Check sheet for the modelled part. Datum: model origin and axes. Units: mm. A direction names the side the tool comes from. Coordinates: 2 decimals unless noted, no trailing zeros. Loops run counter-clockwise (first coordinate to the right, second up) from the corner with the lowest first, then second, coordinate; pieces in that order, holes last. Notation, with made-up numbers: M 43.25,47.5 L 52.25,47.5 A11 ccw 52.25,59.5 Z; hole C 54,37.25 d7. An arc over 180 degrees is marked long. Return JSON: item names as keys, results as strings.
from build123d import *

# Parameters (mm, degrees)
SKETCH_R      = 2.5
PAD_DEPTH     = 65
SKETCH001_W   = 8
SKETCH001_H   = 6
SKETCH001_W_2 = 7
POCKET_DEPTH  = 1.5
CHAMFER_SIZE  = 0.3


with BuildPart() as part:
    # Sketch → Pad (new body)
    with BuildSketch(Plane.YZ):
        Circle(SKETCH_R)
    extrude(amount=PAD_DEPTH)

    # Sketch001 → Pocket (cut)
    with BuildSketch(Plane.XY.offset(3)):
        with Locations((20.5, 0)):
            Rectangle(SKETCH001_W, SKETCH001_H)
        with Locations((45.5, 0)):
            Rectangle(SKETCH001_W_2, SKETCH001_H)
    extrude(amount=-POCKET_DEPTH, mode=Mode.SUBTRACT)

    # Chamfer
    chamfer_edges = [part.edges().sort_by_distance(p)[0] for p in [
        (0, -2.5, 0),
        (65, -2.5, 0),
    ]]
    chamfer(chamfer_edges, length=CHAMFER_SIZE)


solid = part.part
1) Section check B-B on x = 35.5. Record the cut outline in (y, z), then the cut area to 3 significant figures.
Answers:
{"outline": "C 0,0 d5", "area": "19.6 mm²"}
2) Draft check along X on faces 3 (the face through (0, 0, 0)), 4 (the face through (32.05, -0.54, -2.44)), 5 (the face through (24.5, 0, 2)), 6 (the face through (49, 0, 2)). Enter one of: +X half, -X half, draft (parallel to the pull), parting line (faces both ways), or undercut.
Answers:
{"face 3": "-X half", "face 4": "draft", "face 5": "undercut", "face 6": "undercut"}
3) Scan lines: line 1 along X through (y, z) = (-1.3, 1.6); line 2 along Z through (x, y) = (56.5, -0.2); line 3 along Y through (x, z) = (47.5, -1.5). Record each from-to range of solid material in increasing order. Write a range as [from, to].
Answers:
{"line 1": "[0, 16.5], [24.5, 42], [49, 65]", "line 2": "[-2.49, 2.49]", "line 3": "[-2, 2]"}
4) Section check A-A on y = 0. Record the cut outline in (x, z), then the cut area to 3 significant figures.
Answers:
{"outline": "M 0,-2.2 L 0.3,-2.5 L 64.7,-2.5 L 65,-2.2 L 65,2.2 L 64.7,2.5 L 49,2.5 L 49,1.5 L 42,1.5 L 42,2.5 L 24.5,2.5 L 24.5,1.5 L 16.5,1.5 L 16.5,2.5 L 0.3,2.5 L 0,2.2 Z", "area": "310 mm²"}
5) Go/stop test with flat-tipped pins: pin 1 Ø0.8 at (y, z) = (1, 2) entering from -X; pin 2 Ø1.2 at (x, y) = (21.5, 0.5) entering from +Z; pin 3 Ø2 at (x, z) = (9, 1.5) entering from -Y. Record where each tip stops, or that it passes through.
Answers:
{"pin 1": "x = 0", "pin 2": "z = 1.5", "pin 3": "y = -2.45"}
6) Set-up check for faces 1 (the face through (65, 0, 0)), 2 (the face through (45, 0, 1.5)): record each of +Z, -Z, +X, -X, +Y, -Y from which the full face is reachable in a straight line by a thin tool's end or side.
Answers:
{"face 1": "+Z, -Z, +X, +Y, -Y", "face 2": "+Z, +Y, -Y"}
